Part model, mm, in its own coordinate system. Face numbers are marked on the shaded views. Coordinates: 2 decimals unless noted, no trailing zeros. Loops run counter-clockwise (first coordinate to the right, second up) from the corner with the lowest first, then second, coordinate; pieces in that order, holes last.
```python
from build123d import *

# Parameters (mm, degrees)
EXTRUSION1_DEPTH        = 7
ESQUISSE3_R             = 3.375
ENL_V_MAT_EXTRU_1_DEPTH = 8
CHANFREIN1_SIZE         = 1


with BuildPart() as part:
    # Esquisse1 → Extrusion1 (new body)
    with BuildSketch(Plane(origin=(0, 0, 0), x_dir=(0, 0, -1), z_dir=(1, 0, 0))):
        Polygon((0, 8.660254038), (-7.5, 4.330127019), (-7.5, -4.330127019), (0, -8.660254038), (7.5, -4.330127019), (7.5, 4.330127019), align=None)
    extrude(amount=EXTRUSION1_DEPTH)

    # Esquisse2 → Enlèvement de matière-Révolution1 (revolve, cut)
    with BuildSketch(Plane.XY, mode=Mode.PRIVATE) as enl_vement_de_mati_re_r_volution1_sk:
        with BuildLine():
            Line((1.5, 6.75), (1.5, 8.660254038))
            Line((1.5, 8.660254038), (0, 8.660254038))
            Line((0, 8.660254038), (0, 5.25))
            ThreePointArc((0, 5.25), (1.060660172, 5.689339828), (1.5, 6.75))
        make_face()
    revolve(enl_vement_de_mati_re_r_volution1_sk.sketch.rotate(Axis((-3.040359493, 0, 0), (1, 0, 0)), 90), axis=Axis((-3.040359493, 0, 0), (1, 0, 0)), mode=Mode.SUBTRACT)  # turned: the seam where the file's is

    # Esquisse3 → Enlèv. mat.-Extru.1 (cut, through all)
    with BuildSketch(Plane.ZY):
        Circle(ESQUISSE3_R)
    extrude(amount=-ENL_V_MAT_EXTRU_1_DEPTH, mode=Mode.SUBTRACT)

    # Chanfrein1
    chanfrein1_edges = [part.edges().sort_by_distance(p)[0] for p in [
        (7, 0, -3.375),
        (0, 0, -3.375),
    ]]
    chamfer(chanfrein1_edges, length=CHANFREIN1_SIZE)

    # Esquisse4 → Enlèvement de matière-Révolution2 (revolve, cut)
    with BuildSketch(Plane.XY, mode=Mode.PRIVATE) as enl_vement_de_mati_re_r_volution2_sk:
        with BuildLine():
            Line((1.5, 8.660254038), (2.1, 8.660254038))
            ThreePointArc((2.1, 8.660254038), (1.70260937, 8.130490453), (1.5, 7.5))
            Line((1.5, 7.5), (1.5, 8.660254038))
        make_face()
        with BuildLine():
            Line((7, 8.660254038), (7, 7.5))
            ThreePointArc((7, 7.5), (6.79739063, 8.130490453), (6.4, 8.660254038))
            Line((6.4, 8.660254038), (7, 8.660254038))
        make_face()
    revolve(enl_vement_de_mati_re_r_volution2_sk.sketch.rotate(Axis((0, 0, 0), (1, 0, 0)), 270), axis=Axis((0, 0, 0), (1, 0, 0)), mode=Mode.SUBTRACT)  # turned: the seam where the file's is


solid = part.part
```
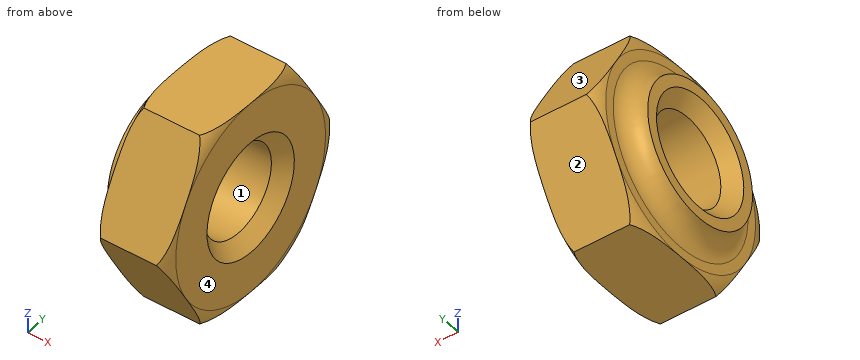
Q1. Saw through at A-A (x = 4.25). List the corners of the cut face in (y, z) (3 decimals), plus the area to 3 significant figures.
Q2. Drop flat-ended pins along their axis: P1, Ø1.5, axis at x = 4.5, z = -5, coming from the -Y side; P2, Ø4, axis at x = 5.5, y = 4.5, coming from the +Z side; P3, Ø6, axis at y = 0, z = 0, coming from the -X side; P4, Ø1, axis at x = 2, z = 3.5, coming from the +Y side. Give the stop position or say it passes through.
Q3. Probe line 1 (X direction, y = 2.5, z = 7); line 2 (Z direction, x = 2, y = 1.5); line 3 (Z direction, x = 0.75, y = -2.75). List the from-to ranges inside material, lowest first.
Q4. Mould opens along Z. For the marked faces 1, 2, 3 and 4 say: released by +Z, released by -Z, zero draft, split by the parting line, or undercut.
Checked values:
1. outline: (-8.66, 0) - (-4.33, -7.5) - (4.33, -7.5) - (8.66, 0) - (4.33, 7.5) - (-4.33, 7.5) - close; hole circle Ø6.75 at (0, 0)
1. area: 159 mm2
2. P1: stops at y = -6.21
2. P2: stops at z = 7.5
2. P3: passes through
2. P4: stops at y = 6.93
3. line 1: x = 1.5 to 7
3. line 2: z = -7.5 to -3.02, 3.02 to 7.5
3. line 3: z = -4.71 to -2.36, 2.36 to 4.71
4. face 1: undercut
4. face 2: released by -Z
4. face 3: released by +Z
4. face 4: zero draft
